Read the model definition and answer for the solid it produces. Units are mm, in the model's axes. A direction names the side the tool comes from. Coordinates: 2 decimals unless noted, no trailing zeros. Write each loop counter-clockwise with the first axis right and the second up, starting at its lowest first coordinate (ties: lowest second). Pieces come first, ordered by that corner, then holes.
Item 1: Section B-B (x = 141) is taken. Give the vertices of the cut face in (y, z) (3 decimals), then the cut area to 3 significant figures.
Item 2: A tool of negligible diameter and unlimited length cuts with its end or side. For faces 5 (the face through (63, 0, 14)), 6 (the face through (41, -31, 11.261)), from which of +Z, -Z, +X, -X, +Y, -Y can it reach the whole face along a straight path? Write none if from no direction.
Item 3: Section D-D (x = 57.5) is taken. Give the vertices of the cut face in (y, z) (3 decimals), then the cut area to 3 significant figures.
Item 4: Each of these flat-tipped pins is pushed along its axis until it touches: P1, Ø16, axis at y = -32.5, z = 37, coming from the +X side; P2, Ø16, axis at y = -24, z = 44, coming from the -X side; P3, Ø12.5, axis at x = 148, y = -27.5, coming from the -Z side. Where does it stop, or does it pass through?
Item 5: Section C-C (z = 57) is taken. Give the vertices of the cut face in (x, y) (3 decimals).
Item 6: Straight lines are drawn through the part: probe 1 along Z at (x, y) = (-8, -4.5); probe 2 along X at (y, z) = (-13.5, 21.5); probe 3 along Z at (x, y) = (131.5, -31.5). For each, find the intervals that lie inside material, in ascending order.
Item 7: Determine the mould class of faces 1 (the face through (63, -62.725, 14)), 2 (the face through (142.6, -39.7, 66.8)), 3 (the face through (41, -31, 14.436)), 4 (the face through (139.33, -19.19, 66.85)) for opening direction Y: released by +Y, released by -Y, zero draft, split by the parting line, or undercut.
Item 8: Section A-A (y = -37) is taken. Give the vertices of the cut face in (x, z).
from build123d import *

# Parameters (mm, degrees)
F0_W     = 3.175
F0_H     = 3.175
F0_W_2   = 25.4
F1_DEPTH = 62.7250036666
F2_R     = 5.08
F3_R     = 2.54
F4_DEPTH = 60.072


with BuildPart() as f1:
    # F0 (on Front) → F1 (new body)
    with BuildSketch(Plane.XZ):
        with BuildLine():
            Line((-47.2060584766, 11.2612042576), (-47.2060584766, 14.4362042576))
            ThreePointArc((-47.2060584766, 14.4362042576), (-47.4333192743, 12.7872299777), (-48.0981569595, 11.2612042576))
            Line((-48.0981569595, 11.2612042576), (-47.2060584766, 11.2612042576))
        make_face()
        Polygon((126.9109415234, 14.4362042576), (-47.2060584766, 14.4362042576), (-47.2060584766, 11.2612042576), (130.0859415234, 11.2612042576), (130.0859415234, 14.4362042576), align=None)
        with BuildLine():
            ThreePointArc((-48.0981569595, 11.2612042576), (-47.4333192743, 12.7872299777), (-47.2060584766, 14.4362042576))
            ThreePointArc((-47.2060584766, 14.4362042576), (-47.4333192743, 16.0851785375), (-48.0981569595, 17.6112042576))
            ThreePointArc((-48.0981569595, 17.6112042576), (-53.3020584766, 20.5322042576), (-58.5059599937, 17.6112042576))
            ThreePointArc((-58.5059599937, 17.6112042576), (-59.3980584766, 14.4362042576), (-58.5059599937, 11.2612042576))
            ThreePointArc((-58.5059599937, 11.2612042576), (-53.3020584766, 8.3402042576), (-48.0981569595, 11.2612042576))
        make_face()
        with BuildLine():
            ThreePointArc((-53.3020584766, 17.4842042576), (-51.1467970075, 16.5914657267), (-50.2540584766, 14.4362042576))
            ThreePointArc((-50.2540584766, 14.4362042576), (-51.1467970075, 12.2809427886), (-53.3020584766, 11.3882042576))
            ThreePointArc((-53.3020584766, 11.3882042576), (-56.3500584766, 14.4362042576), (-53.3020584766, 17.4842042576))
        make_face(mode=Mode.SUBTRACT)
        Polygon((126.9109415234, 68.4112042576), (126.9109415234, 17.6112042576), (130.0859415234, 17.6112042576), (130.0859415234, 65.2362042576), (130.0859415234, 68.4112042576), align=None)
        with Locations((128.4984415234, 16.0237042576)):
            Rectangle(F0_W, F0_H)
        with Locations((142.7859415234, 66.8237042576)):
            Rectangle(F0_W_2, F0_H)
    extrude(amount=F1_DEPTH)

    # F2
    f2_edges = [f1.edges().sort_by_distance(p)[0] for p in [
        (-48.098157, -31.362502, 11.261204),
    ]]
    fillet(f2_edges, radius=F2_R)

    # F3 (on face) → F4 (cut, through all)
    with BuildSketch(Plane.XY.offset(68.4112042576)):
        with Locations((141.1984415234, -20.9083345554)):
            Circle(F3_R)
        with Locations((141.1984415234, -41.8166691112)):
            Circle(F3_R)
    extrude(amount=-F4_DEPTH, mode=Mode.SUBTRACT)


solid = f1.part
Established:
1. outline: (-62.725, 65.236) - (-44.349, 65.236) - (-44.349, 68.411) - (-62.725, 68.411) - close; (-39.284, 65.236) - (-23.441, 65.236) - (-23.441, 68.411) - (-39.284, 68.411) - close; (-18.376, 65.236) - (0, 65.236) - (0, 68.411) - (-18.376, 68.411) - close
1. area: 167 mm2
2. face 5: +Z, -Z, +X, -X, +Y
2. face 6: -Z, +X, +Y, -Y
3. outline: (-62.725, 11.261) - (0, 11.261) - (0, 14.436) - (-62.725, 14.436) - close
3. area: 199 mm2
4. P1: stops at x = 130.09
4. P2: stops at x = 126.91
4. P3: stops at z = 65.24
5. outline: (126.911, -62.725) - (130.086, -62.725) - (130.086, 0) - (126.911, 0) - close
6. probe 1: z = 11.26 to 14.44
6. probe 2: x = 126.91 to 130.09
6. probe 3: z = 65.24 to 68.41
7. face 1: released by -Y
7. face 2: undercut
7. face 3: zero draft
7. face 4: undercut
8. outline: (-49.19, 9.93) arc R5.08 cw to (-45.77, 11.26) - (130.09, 11.26) - (130.09, 65.24) - (155.49, 65.24) - (155.49, 68.41) - (126.91, 68.41) - (126.91, 14.44) - (-47.21, 14.44) arc R6.1 ccw (long way) to start; hole circle Ø6.1 at (-53.3, 14.44)
